Verification items for the finished model (mm, model axes). Give positions to 0.01 mm unless a question says otherwise; leave off trailing zeros. Loops run counter-clockwise (first coordinate to the right, second up) from the corner with the lowest first, then second, coordinate; pieces in that order, holes last. Notation, with made-up numbers: M 6.5,-5.5 L 58.5,-5.5 A16 ccw 58.5,1.5 Z; hole C 5,88 d5. An arc over 180 degrees is marked long. Put each result on its own line as item: value. Start each with the question number.
from build123d import *

# Parameters (mm, degrees)
CROQUIS2_R              = 22.5
SALIENTE_EXTRUIR1_DEPTH = 3


with BuildPart() as part:
    # Croquis2 → Saliente-Extruir1 (new body)
    with BuildSketch(Plane.XY):
        Polygon((-78.032689509, 45.481472081), (-8.032689509, 45.481472081), (-8.032689509, 42.481472081), (1.967310491, 42.481472081), (1.967310491, 45.481472081), (243.967310464, 45.494020393), (243.967310464, 45.480623618), (243.967310464, 42.480623618), (253.967310518, 42.480623618), (253.967310518, 45.480623618), (281.967310491, 45.481472081), (281.967310491, -224.518527919), (211.967310491, -224.548290187), (211.967310491, -221.548290187), (201.967310491, -221.548290187), (201.967310491, -224.548290187), (-40.032689509, -224.518544608), (-40.032689509, -221.518544608), (-50.032689509, -221.518544608), (-50.032689509, -224.518544608), (-78.032689509, -224.518527919), align=None)
        with Locations((-45.032689509, 17.981472081)):
            Circle(CROQUIS2_R, mode=Mode.SUBTRACT)
        with Locations((-45.032689509, -29.518527919)):
            Circle(CROQUIS2_R, mode=Mode.SUBTRACT)
        with Locations((-45.032689509, -77.018527919)):
            Circle(CROQUIS2_R, mode=Mode.SUBTRACT)
        with Locations((-45.032689509, -124.518527919)):
            Circle(CROQUIS2_R, mode=Mode.SUBTRACT)
        with Locations((-45.032689509, -172.018527919)):
            Circle(CROQUIS2_R, mode=Mode.SUBTRACT)
        with Locations((-3.032689509, -5.768527919)):
            Circle(CROQUIS2_R, mode=Mode.SUBTRACT)
        with Locations((38.967310491, 17.981472081)):
            Circle(CROQUIS2_R, mode=Mode.SUBTRACT)
        with Locations((80.967310491, -5.768527919)):
            Circle(CROQUIS2_R, mode=Mode.SUBTRACT)
        with Locations((122.967310491, 17.981472081)):
            Circle(CROQUIS2_R, mode=Mode.SUBTRACT)
        with Locations((164.967310491, -5.768527919)):
            Circle(CROQUIS2_R, mode=Mode.SUBTRACT)
        with Locations((-3.032689509, -53.268527919)):
            Circle(CROQUIS2_R, mode=Mode.SUBTRACT)
        with Locations((-3.032689509, -100.768527919)):
            Circle(CROQUIS2_R, mode=Mode.SUBTRACT)
        with Locations((-3.032689509, -148.268527919)):
            Circle(CROQUIS2_R, mode=Mode.SUBTRACT)
        with Locations((-3.032689509, -195.768527919)):
            Circle(CROQUIS2_R, mode=Mode.SUBTRACT)
        with Locations((37.967310491, -29.518527919)):
            Circle(CROQUIS2_R, mode=Mode.SUBTRACT)
        with Locations((37.967310491, -77.018527919)):
            Circle(CROQUIS2_R, mode=Mode.SUBTRACT)
        with Locations((37.967310491, -124.518527919)):
            Circle(CROQUIS2_R, mode=Mode.SUBTRACT)
        with Locations((37.967310491, -172.018527919)):
            Circle(CROQUIS2_R, mode=Mode.SUBTRACT)
        with Locations((79.967310491, -53.268527919)):
            Circle(CROQUIS2_R, mode=Mode.SUBTRACT)
        with Locations((79.967310491, -100.768527919)):
            Circle(CROQUIS2_R, mode=Mode.SUBTRACT)
        with Locations((79.967310491, -148.268527919)):
            Circle(CROQUIS2_R, mode=Mode.SUBTRACT)
        with Locations((79.967310491, -195.768527919)):
            Circle(CROQUIS2_R, mode=Mode.SUBTRACT)
        with Locations((121.967310491, -29.518527919)):
            Circle(CROQUIS2_R, mode=Mode.SUBTRACT)
        with Locations((163.967310491, -53.268527919)):
            Circle(CROQUIS2_R, mode=Mode.SUBTRACT)
        with Locations((121.967310491, -77.018527919)):
            Circle(CROQUIS2_R, mode=Mode.SUBTRACT)
        with Locations((163.967310491, -100.768527919)):
            Circle(CROQUIS2_R, mode=Mode.SUBTRACT)
        with Locations((121.967310491, -124.518527919)):
            Circle(CROQUIS2_R, mode=Mode.SUBTRACT)
        with Locations((121.967310491, -172.018527919)):
            Circle(CROQUIS2_R, mode=Mode.SUBTRACT)
        with Locations((163.967310491, -148.268527919)):
            Circle(CROQUIS2_R, mode=Mode.SUBTRACT)
        with Locations((163.967310491, -195.768527919)):
            Circle(CROQUIS2_R, mode=Mode.SUBTRACT)
        with Locations((206.967310491, 18.071533546)):
            Circle(CROQUIS2_R, mode=Mode.SUBTRACT)
        with Locations((205.967310491, -29.518527919)):
            Circle(CROQUIS2_R, mode=Mode.SUBTRACT)
        with Locations((205.967310491, -77.018527919)):
            Circle(CROQUIS2_R, mode=Mode.SUBTRACT)
        with Locations((205.967310491, -124.518527919)):
            Circle(CROQUIS2_R, mode=Mode.SUBTRACT)
        with Locations((206.796228515, -171.928466454)):
            Circle(CROQUIS2_R, mode=Mode.SUBTRACT)
        with Locations((248.967310491, -5.768527919)):
            Circle(CROQUIS2_R, mode=Mode.SUBTRACT)
        with Locations((247.967310491, -53.268527919)):
            Circle(CROQUIS2_R, mode=Mode.SUBTRACT)
        with Locations((247.967310491, -100.768527919)):
            Circle(CROQUIS2_R, mode=Mode.SUBTRACT)
        with Locations((247.967310491, -148.268527919)):
            Circle(CROQUIS2_R, mode=Mode.SUBTRACT)
        with Locations((247.967310491, -195.768527919)):
            Circle(CROQUIS2_R, mode=Mode.SUBTRACT)
    extrude(amount=SALIENTE_EXTRUIR1_DEPTH)


solid = part.part
Q1. Cross-section at A-A, the plane x = -44. Record the boundary of the cut face in (y, z).
Q2. Cross-section at B-B, the plane y = -37. State how many separate pieces and enclosed holes the cut face has, then the cut area to 3 significant figures.
Q3. Go/stop test with flat-tipped pins: pin 1 (1 mm diameter, centred on x = 84.5, z = 0.5, fed in from +Y); pin 2 (1.5 mm diameter, centred on x = -2.5, z = 1.5, fed in from +Y). Record where each tip stops, or that it passes through.
Q4. Scan lines: L1, parallel to Y at x = -31, z = 1.95; L2, parallel to Y at x = -51, z = 2.85; L3, parallel to X at y = -208, z = 1.85. Record each from-to range of solid material in increasing order.
Q5. Release check for a two-part mould opening along Y. For faces 1 (the face through (144, -88, 0)), 2 (the face through (-23.57, -70.26, 1.48)), 3 (the face through (77.04, -78.46, 1.48)) record: pulls with the +Y half, pulls with the -Y half, needs draft (parallel to the pull), parting line crosses it, or undercut.
Q6. Cross-section at C-C, the plane x = 250. Record the boundary of the cut face in (y, z), then the cut area to 3 significant figures.
Ans:
1. outline: M -221.52,0 L -194.49,0 L -194.49,3 L -221.52,3 Z; M -149.54,0 L -146.99,0 L -146.99,3 L -149.54,3 Z; M -102.04,0 L -99.49,0 L -99.49,3 L -102.04,3 Z; M -54.54,0 L -51.99,0 L -51.99,3 L -54.54,3 Z; M -7.04,0 L -4.49,0 L -4.49,3 L -7.04,3 Z; M 40.46,0 L 45.48,0 L 45.48,3 L 40.46,3 Z
2. separate pieces: 9
2. enclosed holes: 0
2. area: 198 mm^2
3. pin 1: stops at y = 45.49
3. pin 2: stops at y = 42.48
4. L1: y = -224.52 to -189.61, -154.43 to -142.11, -106.93 to -94.61, -59.43 to -47.11, -11.93 to 0.39, 35.57 to 45.48
4. L2: y = -224.52 to -193.71, -150.32 to -146.21, -102.82 to -98.71, -55.32 to -51.21, -7.82 to -3.71, 39.68 to 45.48
4. L3: x = -78.03 to -21.92, 15.85 to 61.08, 98.85 to 145.08, 182.85 to 229.08, 266.85 to 281.97
5. face 1: needs draft
5. face 2: undercut
5. face 3: undercut
6. outline: M -224.53,0 L -218.18,0 L -218.18,3 L -224.53,3 Z; M -173.36,0 L -170.68,0 L -170.68,3 L -173.36,3 Z; M -125.86,0 L -123.18,0 L -123.18,3 L -125.86,3 Z; M -78.36,0 L -75.68,0 L -75.68,3 L -78.36,3 Z; M -30.86,0 L -28.24,0 L -28.24,3 L -30.86,3 Z; M 16.71,0 L 42.48,0 L 42.48,3 L 16.71,3 Z
6. area: 128 mm^2
